Answer from the drawing. Dimensions are ordinates in mm from the lowest x, y and z of the part. A direction names the side the tool comes from. Give positions to 0.01 mm unless a question says otherwise; leave off trailing zeros. Write each loop counter-clockwise with the first axis right and the second up, starting at its lowest first coordinate (ties: lowest second). Pieces come first, ordered by that corner, then holes. Notation, with made-up numbers: (76, 3.25) - (95, 3.25) arc R8 cw to (95, 10.25) - close; hole circle Ø5 at (-20.5, 1). An arc over 180 degrees is marked (long way). Answer as a JSON object with one key per item and string values. Group by question number.
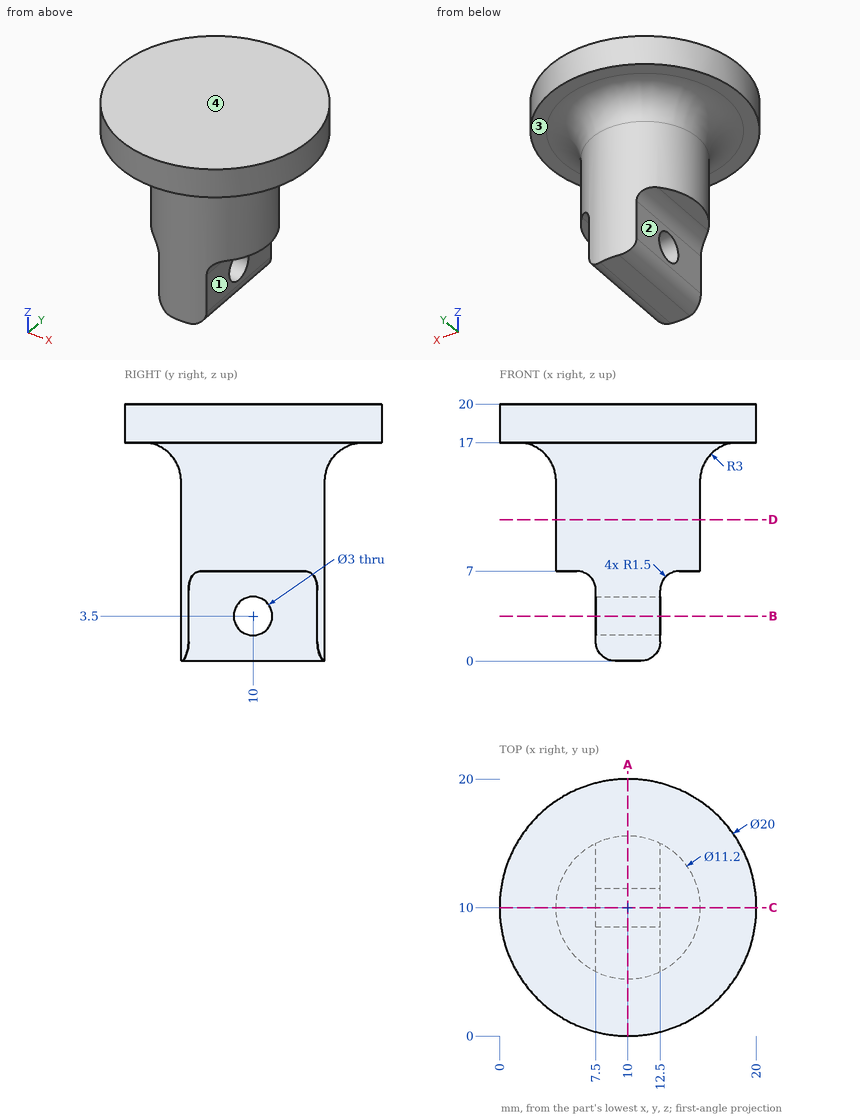
1) Find section A-A, the plane x = 10. Write down the section's boundary in (y, z), and give its area (3 significant figures).
2) Find the intervals of material crossed by line 1 (Y direction, x = 10.15, z = 3.5); line 2 (X direction, y = 6.25, z = 2.5); line 3 (Z direction, x = 19, y = 7.75), in increasing order. Write a range as [from, to].
3) Which of the six approach directions +Z, -Z, +X, -X, +Y, -Y give full straight-line access (tool end or side, diameter ignored) to the marked faces 1, 2, 3 and 4?
4) Flat-ended cylindrical pins translate along their axes: pin 1 Ø1.5 at (y, z) = (17.5, 11) entering from -X; pin 2 Ø5 at (y, z) = (14.5, 12) entering from +X; pin 3 Ø0.8 at (x, y) = (15, 11.5) entering from -Z; pin 4 Ø3 at (x, z) = (7, 17.5) entering from -Y. Find the tip coordinate at first contact, or state that the pin passes through.
5) Find section D-D, the plane z = 11. Write down the section's boundary in (x, y), and give its area (3 significant figures).
6) Find section B-B, the plane z = 3.5. Write down the section's boundary in (x, y), and give its area (3 significant figures).
7) Find section C-C, the plane y = 10. Write down the section's boundary in (x, z), and give its area (3 significant figures).
Values follow:
{
 "1": {"outline": "(0, 17) - (1.4, 17) arc R3 cw to (4.4, 14) - (4.4, 0) - (15.6, 0) - (15.6, 14) arc R3 cw to (18.6, 17) - (20, 17) - (20, 20) - (0, 20) - close; hole circle Ø3 at (10, 3.5)", "area": "247 mm2"},
 "2": {"line 1": "y = [4.4, 8.5], [11.5, 15.6]", "line 2": "x = [7.5, 12.5]", "line 3": "z = [17, 20]"},
 "3": {"face 1": "-Z, +X, +Y, -Y", "face 2": "-Z, -X, +Y, -Y", "face 3": "-Z", "face 4": "+Z, +X, -X, +Y, -Y"},
 "4": {"pin 1": "passes through", "pin 2": "stops at x = 15.23", "pin 3": "stops at z = 7", "pin 4": "stops at y = 0.11"},
 "5": {"outline": "circle Ø11.2 at (10, 10)", "area": "98.5 mm2"},
 "6": {"outline": "(7.5, 4.99) arc R5.6 ccw to (12.5, 4.99) - (12.5, 8.5) - (7.5, 8.5) - close; (7.5, 11.5) - (12.5, 11.5) - (12.5, 15.01) arc R5.6 ccw to (7.5, 15.01) - close", "area": "39.1 mm2"},
 "7": {"outline": "(0, 17) - (1.4, 17) arc R3 cw to (4.4, 14) - (4.4, 7) - (6, 7) arc R1.5 cw to (7.5, 5.5) - (7.5, 5) - (12.5, 5) - (12.5, 5.5) arc R1.5 cw to (14, 7) - (15.6, 7) - (15.6, 14) arc R3 cw to (18.6, 17) - (20, 17) - (20, 20) - (0, 20) - close; (7.5, 1.5) arc R1.5 ccw to (9, 0) - (11, 0) arc R1.5 ccw to (12.5, 1.5) - (12.5, 2) - (7.5, 2) - close", "area": "196 mm2"}
}
